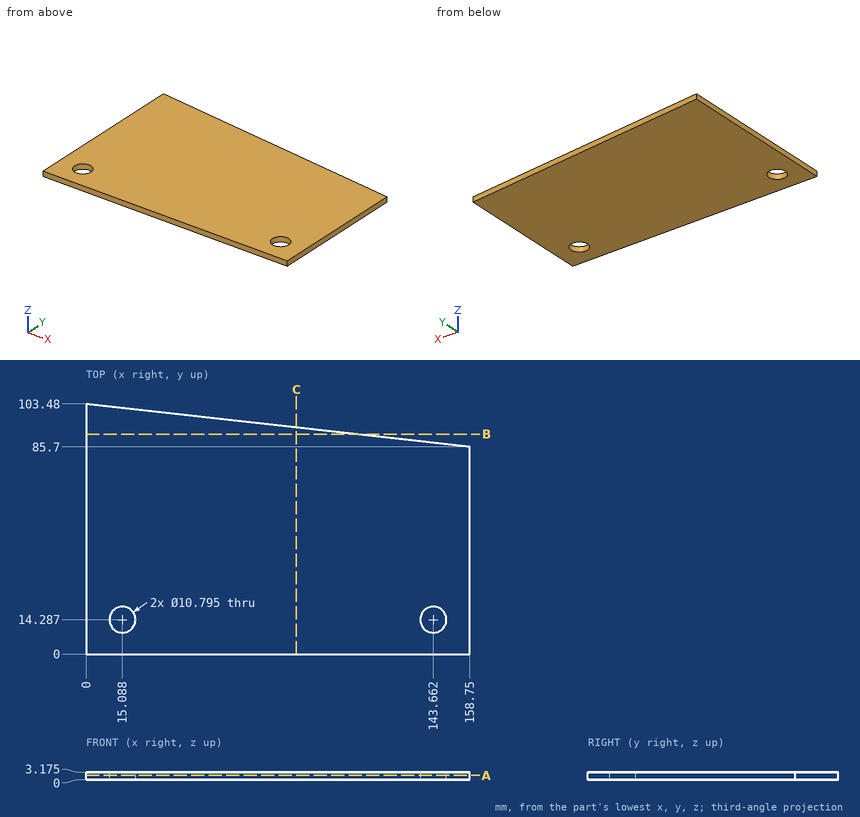
Answer from the drawing. Dimensions are ordinates in mm from the lowest x, y and z of the part. Round coordinates to 2 decimals unless told otherwise and drop trailing zeros. Write each loop counter-clockwise with the first axis right and the second up, starting at its lowest first coordinate (ties: lowest second). Pieces come first, ordered by that corner, then holes.
1. Straight lines are drawn through the part: L1, parallel to Y at x = 143, z = 0.9 (1 decimal); L2, parallel to Y at x = 85, z = 0.1; L3, parallel to Y at x = 51, z = 3.05. For each, find the intervals that lie inside material, in ascending order.
2. The part is cut by section A-A, the plane z = 1.85. State how many separate pieces and enclosed holes the cut face has, then the cut area to 3 significant figures.
3. The part is cut by section C-C, the plane x = 87. Determine the outline of the cut face in (y, z) (1 decimal).
4. The part is cut by section B-B, the plane y = 91. Determine the outline of the cut face in (x, z) (1 decimal).
Values:
1. L1: y = 0 to 8.9, 19.6 to 87.5
1. L2: y = 0 to 93.96
1. L3: y = 0 to 97.77
2. separate pieces: 1
2. enclosed holes: 2
2. area: 14,800 mm2
3. outline: (0, 0) - (93.7, 0) - (93.7, 3.2) - (0, 3.2) - close
4. outline: (0, 0) - (111.4, 0) - (111.4, 3.2) - (0, 3.2) - close
